Study the drawing (mm; zero at the part's minimum x, y, z) and answer. A direction names the side the tool comes from. Coordinates: 2 decimals unless noted, no trailing zeros. Write each loop counter-clockwise with the first axis right and the second up, starting at its lowest first coordinate (ties: lowest second). Pieces come first, ordered by that corner, then holes. Notation, with made-up numbers: (48, 27) -> (65, 27) arc R30 cw to (65, 51) -> close; hole circle Ø1 at (48, -12.75). An arc over 180 degrees is marked (long way). Answer in a Markdown table with one row per item. Add a question column.
Item 1: Which of the six approach directions +Z, -Z, +X, -X, +Y, -Y give full straight-line access (tool end or side, diameter ignored) to the marked faces 1 and 2?
Item 2: Section B-B on x = 38.5 is taken. Write down the section's boundary in (y, z).
Item 3: Straight lines are drawn through the part: line 1 (Y direction, x = 60.5, z = 29); line 2 (Y direction, x = 8, z = 17) (1 decimal). For each, find the intervals that lie inside material, in ascending order. Write a range as from..to.
Item 4: Given pin 1 Ø8 at (y, z) = (16.5, 27.5) entering from +X; pin 2 Ø24 at (y, z) = (31.5, 26.5) entering from +X; pin 3 Ø20 at (x, z) = (48, 28.5) entering from +Y, each flat-ended and moving along its own axis, determine where each tip first touches the part or whether it passes through.
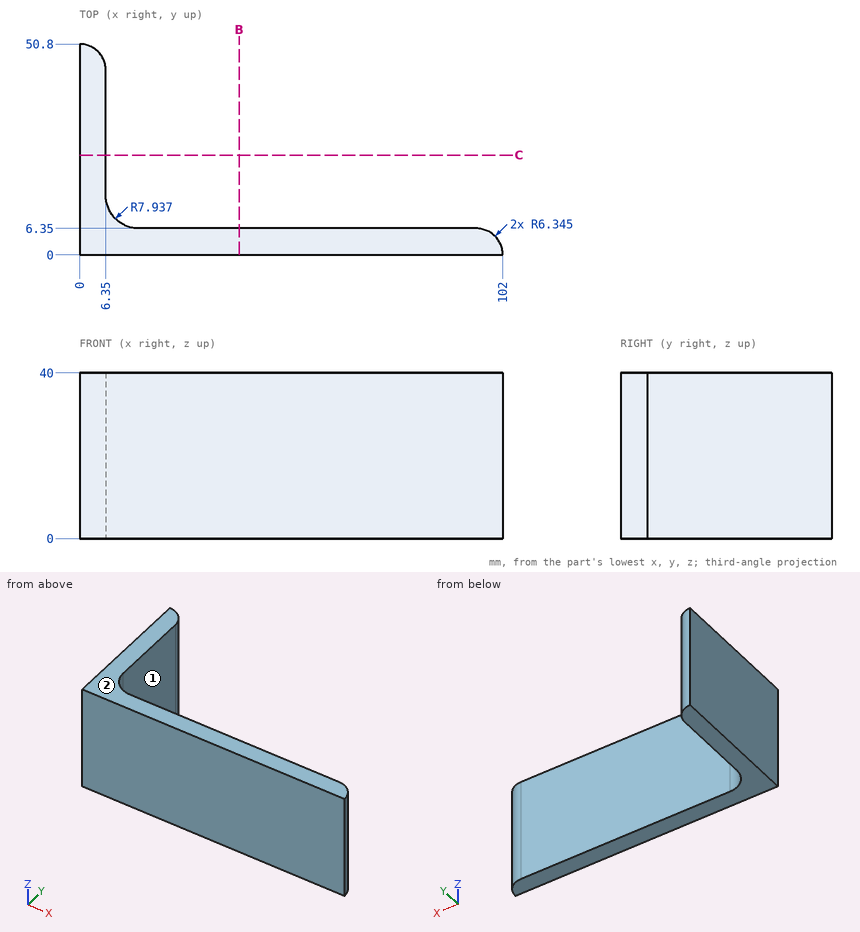
Results below:
| question | item | result |
|---|---|---|
| 1 | face 1 | +Z, -Z, +X, +Y |
| 1 | face 2 | +Z, +X, -X, +Y, -Y |
| 2 | outline | (0, 0) -> (6.35, 0) -> (6.35, 40) -> (0, 40) -> close |
| 3 | line 1 | y = 0..6.35 |
| 3 | line 2 | y = 0..9.4 |
| 4 | pin 1 | stops at x = 6.55 |
| 4 | pin 2 | stops at x = 6.35 |
| 4 | pin 3 | stops at y = 6.35 |
